CAD build for the part. Positions are in the model's coordinates, mm. A direction names the side the tool comes from. Coordinates: 2 decimals unless noted, no trailing zeros. Loops run counter-clockwise (first coordinate to the right, second up) from the corner with the lowest first, then second, coordinate; pieces in that order, holes last.
1) Saw through at B-B, the plane x = -43.5. Write the cut outline in (y, z), and give its area (3 significant figures).
2) Pin check, flat tips, straight feed: pin 1 Ø6 at (x, z) = (-36, -7) entering from +Y; pin 2 Ø4.5 at (x, y) = (-29.5, 5.5) entering from -Z; pin 3 Ø5 at (y, z) = (9.5, -8) entering from +X. Stop position of each tip, or through.
3) Two-plate mould, pull along X, no slides. Class faces 5 (the flat face through (-45.197, 9, -2)), 6 (the flat face through (-21.947, 7, -39)), 7 (the flat face through (-30, 7, 23.456)): +X half, -X half, draft (parallel to the pull), parting line (faces both ways), or undercut.
4) Saw through at A-A, the plane z = -2. Write the cut outline in (x, y), and give its area (3 significant figures).
5) Wall check: line 1 along Z through (x, y) = (17.5, 7); line 2 along Z through (x, y) = (10, 13.5); line 3 along X through (y, z) = (10.5, 11). Give the ranges that are in metal, low to high.
6) Which spindle directions (+Z, -Z, +X, -X, +Y, -Y) get a long thin tool onto all of the face, cutting with end or side? Do faces 1 (the flat face through (-33, 3, -27.544)), 2 (the flat face through (21, 14.418, 13)), 3 (the flat face through (-39, 4, -2)), 4 (the flat face through (-21.947, 7, 35)). Say none if no direction does.
```python
from build123d import *

# Parameters (mm, degrees)
SKETCH1_W           = 95
SKETCH1_H           = 95
BOSS_EXTRUDE1_DEPTH = 50
CUT_EXTRUDE1_DEPTH  = 100
SKETCH3_R           = 9.5
CUT_EXTRUDE2_DEPTH  = 45
CUT_EXTRUDE4_DEPTH  = 45
CUT_EXTRUDE5_DEPTH  = 45
CUT_EXTRUDE6_DEPTH  = 45
CUT_EXTRUDE7_DEPTH  = 45
SKETCH9_R           = 9.5
CUT_EXTRUDE9_DEPTH  = 45
SKETCH11_R          = 9.5
CUT_EXTRUDE10_DEPTH = 45
SKETCH12_W          = 31.985759797
SKETCH12_H          = 95
BOSS_EXTRUDE2_DEPTH = 45
CUT_EXTRUDE11_DEPTH = 100
SKETCH14_R          = 9.5
CUT_EXTRUDE12_DEPTH = 100
SKETCH15_R          = 9.5
CUT_EXTRUDE13_DEPTH = 100
SKETCH16_R          = 9.5
CUT_EXTRUDE14_DEPTH = 100
FILLET2_R           = 4
SKETCH17_W          = 34
SKETCH17_H          = 34
CUT_EXTRUDE16_DEPTH = 22
SKETCH19_W          = 34
SKETCH19_H          = 34
CUT_EXTRUDE17_DEPTH = 22
SKETCH20_W          = 12.5
SKETCH20_H          = 16.5
CUT_EXTRUDE18_DEPTH = 60
CUT_EXTRUDE19_DEPTH = 60
CUT_EXTRUDE20_DEPTH = 100


with BuildPart() as part:
    # Sketch1 → Boss-Extrude1 (new body)
    with BuildSketch(Plane(origin=(0, 0, 0), x_dir=(1, 0, 0), z_dir=(0, 1, 0))):
        with Locations((-8.446550514, 2.043801884)):
            Rectangle(SKETCH1_W, SKETCH1_H)
    extrude(amount=BOSS_EXTRUDE1_DEPTH)

    # Sketch2 → Cut-Extrude1 (cut)
    with BuildSketch(Plane.XY.offset(45.456198116)):
        Polygon((39.053449486, 0), (36.353449486, 50), (39.053449486, 50), align=None)
    extrude(amount=-CUT_EXTRUDE1_DEPTH, mode=Mode.SUBTRACT)

    # Sketch3 → Cut-Extrude2 (cut)
    with BuildSketch(Plane(origin=(38.939900735, 2.10275464, 0), x_dir=(0, 0, -1), z_dir=(0.998545181, 0.05392144, 0))):
        with Locations((2.043801884, 13.394181776)):
            Circle(SKETCH3_R)
    extrude(amount=-CUT_EXTRUDE2_DEPTH, mode=Mode.SUBTRACT)

    # Sketch5 → Cut-Extrude4 (cut)
    with BuildSketch(Plane(origin=(0, 50, 0), x_dir=(1, 0, 0), z_dir=(0, 1, 0))):
        Polygon((39.053449486, 49.543801884), (39.053449486, 29.543801884), (19.053449486, 49.543801884), align=None)
        Polygon((39.053449486, -45.456198116), (39.053449486, -25.456198116), (19.053449486, -45.456198116), align=None)
    extrude(amount=-CUT_EXTRUDE4_DEPTH, mode=Mode.SUBTRACT)

    # Sketch6 → Cut-Extrude5 (cut)
    with BuildSketch(Plane(origin=(0, 50, 0), x_dir=(1, 0, 0), z_dir=(0, 1, 0))):
        Polygon((19.053449486, -45.456198116), (12.925569587, -39.328318218), (6.797689689, -45.456198116), align=None)
        Polygon((19.053449486, 49.543801884), (12.925569587, 43.415921985), (6.797689689, 49.543801884), align=None)
    extrude(amount=-CUT_EXTRUDE5_DEPTH, mode=Mode.SUBTRACT)

    # Sketch7 → Cut-Extrude6 (cut)
    with BuildSketch(Plane(origin=(-13.201374315, 0, 13.201374315), x_dir=(0.707106781, 0, 0.707106781), z_dir=(-0.707106781, 0, 0.707106781))):
        Polygon((45.615209271, 5), (42.915209271, 50), (45.615209271, 50), align=None)
    extrude(amount=-CUT_EXTRUDE6_DEPTH, mode=Mode.SUBTRACT)

    # Sketch8 → Cut-Extrude7 (cut)
    with BuildSketch(Plane(origin=(-15.245176199, 0, -15.245176199), x_dir=(-0.707106781, 0, 0.707106781), z_dir=(-0.707106781, 0, -0.707106781))):
        Polygon((-48.505581614, 5), (-45.805581614, 50), (-48.505581614, 50), align=None)
    extrude(amount=-CUT_EXTRUDE7_DEPTH, mode=Mode.SUBTRACT)

    # Sketch9 → Cut-Extrude9 (cut)
    with BuildSketch(Plane(origin=(34.386964646, 2.917830706, -34.386964646), x_dir=(-0.708373873, 0.059677836, -0.70331004), z_dir=(0.705837415, 0.059892291, -0.705837415))):
        with Locations((14.526974541, 11.311121921)):
            Circle(SKETCH9_R)
    extrude(amount=-CUT_EXTRUDE9_DEPTH, mode=Mode.SUBTRACT)

    # Sketch11 → Cut-Extrude10 (cut)
    with BuildSketch(Plane(origin=(32.350494057, 2.745030447, 32.350494057), x_dir=(0.70331004, 0.059677836, -0.708373873), z_dir=(0.705837415, 0.059892291, 0.705837415))):
        with Locations((-10.17752107, 12.964151979)):
            Circle(SKETCH11_R)
    extrude(amount=-CUT_EXTRUDE10_DEPTH, mode=Mode.SUBTRACT)

    # Sketch12 → Boss-Extrude2 (add)
    with BuildSketch(Plane(origin=(0, 5, 0), x_dir=(1, 0, 0), z_dir=(0, 1, 0))):
        with Locations((22.790569588, 2.043801884)):
            Rectangle(SKETCH12_W, SKETCH12_H)
    extrude(amount=BOSS_EXTRUDE2_DEPTH)

    # Sketch13 → Cut-Extrude11 (cut)
    with BuildSketch(Plane.XY.offset(45.456198116)):
        Polygon((39.053449486, 0), (29.053449486, 3), (19.053449486, 50), (49.745275601, 50), align=None)
    extrude(amount=-CUT_EXTRUDE11_DEPTH, mode=Mode.SUBTRACT)

    # Sketch14 → Cut-Extrude12 (cut)
    with BuildSketch(Plane(origin=(-5.994632406, -0.32371015, 0), x_dir=(0, 0, -1), z_dir=(0.998545181, 0.05392144, 0))):
        with Locations((2.043801884, 13.394181776)):
            Circle(SKETCH14_R)
    extrude(amount=CUT_EXTRUDE12_DEPTH, mode=Mode.SUBTRACT)

    # Sketch15 → Cut-Extrude13 (cut)
    with BuildSketch(Plane(origin=(0.587810371, 0.049877364, 0.587810371), x_dir=(0.70331004, 0.059677836, -0.708373873), z_dir=(0.705837415, 0.059892291, 0.705837415))):
        with Locations((-10.17752107, 12.964151979)):
            Circle(SKETCH15_R)
    extrude(amount=CUT_EXTRUDE13_DEPTH, mode=Mode.SUBTRACT)

    # Sketch16 → Cut-Extrude14 (cut)
    with BuildSketch(Plane(origin=(2.62428096, 0.222677624, -2.62428096), x_dir=(-0.708373873, 0.059677836, -0.70331004), z_dir=(0.705837415, 0.059892291, -0.705837415))):
        with Locations((14.526974541, 11.311121921)):
            Circle(SKETCH16_R)
    extrude(amount=CUT_EXTRUDE14_DEPTH, mode=Mode.SUBTRACT)

    # Fillet2
    fillet2_edges = [part.edges().sort_by_distance(p)[0] for p in [
        (29.053449486, 3, -2.043801884),
    ]]
    fillet(fillet2_edges, radius=FILLET2_R)

    # Sketch17 → Cut-Extrude16 (cut)
    with BuildSketch(Plane.XY.offset(45.456198116)):
        with Locations((-38.946550514, 17)):
            Rectangle(SKETCH17_W, SKETCH17_H)
    extrude(amount=-CUT_EXTRUDE16_DEPTH, mode=Mode.SUBTRACT)

    # Sketch19 → Cut-Extrude17 (cut)
    with BuildSketch(Plane(origin=(0, 0, -49.543801884), x_dir=(-1, 0, 0), z_dir=(0, 0, -1))):
        with Locations((38.946550514, 17)):
            Rectangle(SKETCH19_W, SKETCH19_H)
    extrude(amount=-CUT_EXTRUDE17_DEPTH, mode=Mode.SUBTRACT)

    # Sketch20 → Cut-Extrude18 (cut)
    with BuildSketch(Plane.XY.offset(23.456198116)):
        with Locations((-38.946550514, 12.25)):
            Rectangle(SKETCH20_W, SKETCH20_H)
    extrude(amount=-CUT_EXTRUDE18_DEPTH, mode=Mode.SUBTRACT)

    # Sketch21 → Cut-Extrude19 (cut)
    with BuildSketch(Plane.XY.offset(23.456198116)):
        Polygon((-55.946550514, 34), (-48.446550514, 0), (-55.946550514, 0), align=None)
    extrude(amount=-CUT_EXTRUDE19_DEPTH, mode=Mode.SUBTRACT)

    # Sketch22 → Cut-Extrude20 (cut)
    with BuildSketch(Plane.XY.offset(45.456198116)):
        Polygon((16.581652311, 14.417739075), (-57.762384818, 14.417739075), (-57.762384818, 55.877932289), (42.054048577, 55.877932289), (42.054048577, 14.417739075), align=None)
    extrude(amount=-CUT_EXTRUDE20_DEPTH, mode=Mode.SUBTRACT)


solid = part.part
```
Data:
1. outline: (0, -27.54) - (4, -27.54) - (4, 23.46) - (0, 23.46) - close
1. area: 204 mm2
2. pin 1: stops at y = 4
2. pin 2: stops at z = -27.54
2. pin 3: stops at x = 28.2
3. face 5: undercut
3. face 6: -X half
3. face 7: draft
4. outline: (-51.63, 14.42) - (-48.45, 0) - (39.05, 0) - (31.32, 2.32) arc R4 cw to (28.56, 5.32) - (28.53, 5.44) - (-6.2, 3.56) - (-6.79, 14.42) - (-32.7, 14.42) - (-32.7, 4) - (-45.2, 4) - (-45.2, 14.42) - close
4. area: 673 mm2
5. line 1: z = -49.54 to -44.71, -28.13 to -8.07, 3.98 to 24.04, 40.62 to 45.46
5. line 2: z = -49.54 to -42.92, -16.12 to -11.53, 7.45 to 12.03, 38.83 to 45.46
5. line 3: x = -50.76 to -45.2, -32.7 to -10.71, 8.43 to 27.46
6. face 1: -Z, -X, +Y, -Y
6. face 2: +Z, -Z, +X, -X, +Y
6. face 3: +Z, -Z, +Y
6. face 4: +Z, -X, +Y, -Y
